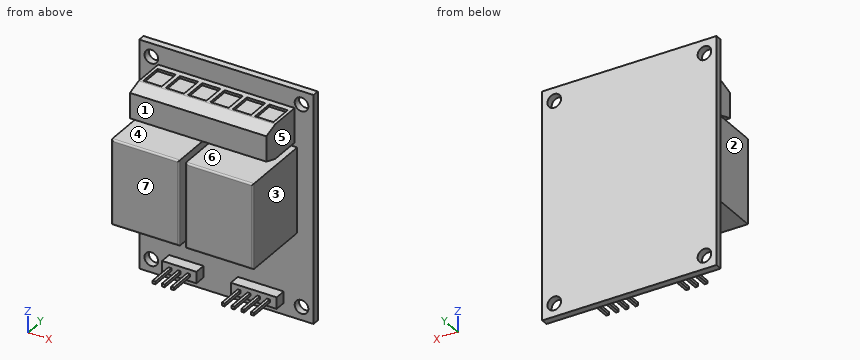
from build123d import *

# Parameters (mm, degrees)
F0_W      = 38.608
F0_H      = 50.419
F0_R      = 1.5113
F1_DEPTH  = 1.524
F2_W      = 14.986
F2_H      = 18.796
F3_DEPTH  = 15.875
F4_R      = 0.381
F5_W      = 30.226
F5_H      = 7.62
F6_DEPTH  = 10.16
F7_SIZE2  = 1.016
F7_SIZE   = 3.175
F8_W      = 4.064
F8_H      = 5.08
F9_DEPTH  = 0.508
F10_W     = 7.62
F10_H     = 2.54
F10_W_2   = 10.16
F11_DEPTH = 2.54
F12_W     = 0.635
F12_H     = 0.635
F13_DEPTH = 5.715


with BuildPart() as f1:
    # F0 (on Front) → F1 (new body)
    with BuildSketch(Plane.XZ):
        Rectangle(F0_W, F0_H)
        with Locations((-16.637, -22.2885)):
            Circle(F0_R, mode=Mode.SUBTRACT)
        with Locations((16.637, -22.2885)):
            Circle(F0_R, mode=Mode.SUBTRACT)
        with Locations((-16.637, 22.2885)):
            Circle(F0_R, mode=Mode.SUBTRACT)
        with Locations((16.637, 22.2885)):
            Circle(F0_R, mode=Mode.SUBTRACT)
    extrude(amount=F1_DEPTH)

    # F2 (on face) → F3 (join)
    with BuildSketch(Plane.XZ.offset(1.524)):
        with Locations((-8.1915, 3.1115)):
            Rectangle(F2_W, F2_H)
        with Locations((8.1915, 3.1115)):
            Rectangle(F2_W, F2_H)
    extrude(amount=F3_DEPTH)

    # F4
    f4_edges = [f1.edges().sort_by_distance(p)[0] for p in [
        (-8.1915, -17.399, 12.5095),
        (-15.6845, -17.399, 3.1115),
        (-8.1915, -17.399, -6.2865),
        (-0.6985, -17.399, 3.1115),
        (0.6985, -17.399, 3.1115),
        (8.1915, -17.399, -6.2865),
        (15.6845, -17.399, 3.1115),
        (8.1915, -17.399, 12.5095),
    ]]
    fillet(f4_edges, radius=F4_R)

    # F5 (on face) → F6 (join)
    with BuildSketch(Plane.XZ.offset(1.524)):
        with Locations((0, 17.2085)):
            Rectangle(F5_W, F5_H)
    extrude(amount=F6_DEPTH)

    # F7
    f7_edges = [f1.edges().sort_by_distance(p)[0] for p in [
        (0, -11.684, 21.0185),
        (0, -11.684, 13.3985),
    ]]
    chamfer(f7_edges, length=F7_SIZE, length2=F7_SIZE2)

    # F8 (on face) → F9 (cut)
    with BuildSketch(Plane.XY.offset(21.0185)):
        with Locations((-12.3825, -5.461)):
            Rectangle(F8_W, F8_H)
        with Locations((-7.4295, -5.461)):
            Rectangle(F8_W, F8_H)
        with Locations((-2.4765, -5.461)):
            Rectangle(F8_W, F8_H)
        with Locations((2.4765, -5.461)):
            Rectangle(F8_W, F8_H)
        with Locations((7.4295, -5.461)):
            Rectangle(F8_W, F8_H)
        with Locations((12.3825, -5.461)):
            Rectangle(F8_W, F8_H)
    extrude(amount=-F9_DEPTH, mode=Mode.SUBTRACT)

    # F10 (on face) → F11 (join)
    with BuildSketch(Plane.XZ.offset(1.524)):
        with Locations((-8.89, -21.3995)):
            Rectangle(F10_W, F10_H)
        with Locations((7.62, -21.3995)):
            Rectangle(F10_W_2, F10_H)
    extrude(amount=F11_DEPTH)

    # F12 (on face) → F13 (join)
    with BuildSketch(Plane.XZ.offset(4.064)):
        with Locations((4.3815, -21.3995)):
            Rectangle(F12_W, F12_H)
        with Locations((6.5405, -21.3995)):
            Rectangle(F12_W, F12_H)
        with Locations((8.6995, -21.3995)):
            Rectangle(F12_W, F12_H)
        with Locations((10.8585, -21.3995)):
            Rectangle(F12_W, F12_H)
        with Locations((-6.82625, -21.3995)):
            Rectangle(F12_W, F12_H)
        with Locations((-8.89, -21.3995)):
            Rectangle(F12_W, F12_H)
        with Locations((-10.95375, -21.3995)):
            Rectangle(F12_W, F12_H)
    extrude(amount=F13_DEPTH)


solid = f1.part
The listing builds one solid part. Answer for the finished solid, in the listing's coordinates (mm). Face numbers are marked on the shaded views. A direction names the side the tool comes from. Coordinates: 2 decimals unless noted, no trailing zeros. Order: outer loops, then holes, each group sorted by start corner. A loop starts at its lowest first (then second) coordinate and runs counter-clockwise, first axis right, second up. Notation, with made-up numbers: (-16, 65.25) -> (4, 65.25) arc R29 cw to (4, 91.25) -> close; hole circle Ø9 at (65, -38.75). An arc over 180 degrees is marked (long way). Answer in a Markdown table with one row per item. Add a question column.
Item 1: Find section A-A (y = -15.5). Write down the section's boundary in (x, z), then the cut area to 3 significant figures.
Item 2: Find the intervals of material crossed by L1, parallel to Z at x = 8, y = -3.5; L2, parallel to Z at x = -15, y = -6.5; L3, parallel to X at y = -16, z = 11, in increasing order. Write a range as from..to.
Item 3: Each of these flat-tipped pins is pushed along its axis until it touches: P1, Ø4, axis at x = -5.5, z = -8, coming from the +Y side; P2, Ø8, axis at y = -12.5, z = 6, coming from the +X side; P3, Ø1.3, axis at y = -2.5, z = -21.5, coming from the +X side; P4, Ø2, axis at x = 5.5, y = -5, coming from the -Z side. Where does it stop, or does it pass through?
Item 4: Find section C-C (x = -3). Write down the section's boundary in (y, z), then the cut area to 3 significant figures.
Item 5: Determine the mould class of the marked faces 6 and 7 for opening direction Z: +Z half, -Z half, draft (parallel to the pull), parting line (faces both ways), or undercut.
Item 6: Find section B-B (z = 16). Write down the section's boundary in (x, y).
Item 7: Which of the six approach directions +Z, -Z, +X, -X, +Y, -Y give full straight-line access (tool end or side, diameter ignored) to the marked faces 1, 2, 3, 4 and 5?
Item 8: Find section D-D (x = 17.5). Write down the section's boundary in (y, z), then the cut area to 3 significant figures.
Result set:
| question | item | result |
|---|---|---|
| 1 | outline | (-15.68, -6.29) -> (-0.7, -6.29) -> (-0.7, 12.51) -> (-15.68, 12.51) -> close; (0.7, -6.29) -> (15.68, -6.29) -> (15.68, 12.51) -> (0.7, 12.51) -> close |
| 1 | area | 563 mm² |
| 2 | L1 | z = -22.67..-20.13, -6.29..12.51, 13.4..20.51 |
| 2 | L2 | z = -6.29..12.51, 13.4..21.02 |
| 2 | L3 | x = -15.68..-0.7, 0.7..15.68 |
| 3 | P1 | stops at y = 0 |
| 3 | P2 | stops at x = 15.68 |
| 3 | P3 | stops at x = 12.7 |
| 3 | P4 | stops at z = -22.67 |
| 4 | outline | (-17.4, -5.91) arc R0.38 ccw to (-17.02, -6.29) -> (-1.52, -6.29) -> (-1.52, -25.21) -> (0, -25.21) -> (0, 25.21) -> (-1.52, 25.21) -> (-1.52, 21.02) -> (-2.92, 21.02) -> (-2.92, 20.51) -> (-8, 20.51) -> (-8, 21.02) -> (-8.51, 21.02) -> (-11.68, 20) -> (-11.68, 14.41) -> (-8.51, 13.4) -> (-1.52, 13.4) -> (-1.52, 12.51) -> (-17.02, 12.51) arc R0.38 ccw to (-17.4, 12.13) -> close |
| 4 | area | 447 mm² |
| 5 | face 6 | undercut |
| 5 | face 7 | draft |
| 6 | outline | (-19.3, -1.52) -> (-15.11, -1.52) -> (-15.11, -11.68) -> (15.11, -11.68) -> (15.11, -1.52) -> (19.3, -1.52) -> (19.3, 0) -> (-19.3, 0) -> close |
| 7 | face 1 | +Z, +X, -X, -Y |
| 7 | face 2 | +Z, -Z, -X, -Y |
| 7 | face 3 | +Z, -Z, +X, -Y |
| 7 | face 4 | +X, -X, -Y |
| 7 | face 5 | +Z, +X, -Y |
| 8 | outline | (-1.52, -25.21) -> (0, -25.21) -> (0, -23.53) -> (-1.52, -23.53) -> close; (-1.52, -21.05) -> (0, -21.05) -> (0, 21.05) -> (-1.52, 21.05) -> close; (-1.52, 23.53) -> (0, 23.53) -> (0, 25.21) -> (-1.52, 25.21) -> close |
| 8 | area | 69.3 mm² |
